Geometry check sheet. Reference: the model listing, model coordinates, mm. A direction names the side the tool comes from. Give positions to 0.01 mm unless a question says otherwise; leave off trailing zeros. Write each loop counter-clockwise with the first axis right and the second up, starting at its lowest first coordinate (ties: lowest second). Pieces come first, ordered by that corner, then holes.
(1) Cross-section at C-C (y = 1.25). Record the boundary of the cut face in (x, z).
(2) Mould release check, pull along Z, two halves, no side actions. Record for faces 1 (the flat face through (-2, 9, 5)), 2 (the cylindrical face through (-7.81, 12.99, -1.73)), 3 (the flat face through (-6, 0, 6)): +Z half, -Z half, draft (parallel to the pull), parting line (faces both ways), or undercut.
(3) Cross-section at B-B (z = 0). Record the boundary of the cut face in (x, y).
(4) Cross-section at A-A (x = 0). Record the boundary of the cut face in (y, z).
(5) Cross-section at D-D (x = 12.5). Record the boundary of the cut face in (y, z).
(6) Tool access check on faces 4 (the cylindrical face through (-4.88, 12.45, -1.08)), 5 (the cylindrical face through (-9.76, 14.49, -2.17)), 6 (the flat face through (8.2, 14, 0)), 7 (the cylindrical face through (0.33, 4.437, -7.493)). Record the directions out of +Z, -Z, +X, -X, +Y, -Y that give a thin tool (end or side, any length) a straight path to the whole face; none if there is none.
(7) Depth check by flat-ended pin: P1, Ø12, axis at x = -3.5, z = 1, coming from the -Y side; P2, Ø1.5, axis at x = 8.5, z = -9.5, coming from the +Y side; P3, Ø4, axis at x = 1, z = 1, coming from the -Y side; P4, Ø6, axis at y = 7.5, z = 9.5, coming from the -X side. Enter the tip coordinate at first touch or a pass-through.
(8) Thickness scan on line 1 along X through (y, z) = (11.5, 0); line 2 along X through (y, z) = (4, 0); line 3 along Y through (x, z) = (-2.5, -7.75). Record the ranges inside material, lowest first.
```python
from build123d import *

# Parameters (mm, degrees)
SKETCH_1_R           = 14.5
SKETCH_1_R_2         = 7.5
EXTRUDE_1_DEPTH      = 12
EXTRUDE_2_DEPTH      = 2
EXTRUDE_2_DEPTH_BACK = 3
SKETCH_2_R           = 8
SKETCH_2_R_2         = 5
SKETCH_3_R           = 10
SKETCH_3_R_2         = 5
EXTRUDE_3_DEPTH      = 2
FILLET_1_R           = 1


with BuildPart() as part:
    # Эскиз1 → Бобышка-Вытянуть1 (new body)
    with BuildSketch(Plane(origin=(0, 0, 0), x_dir=(1, 0, 0), z_dir=(0, 1, 0))):
        with Locations(Location((0, 0, 0), (0, 0, 270))):
            Circle(SKETCH_1_R)
        with Locations(Location((0, 0, 0), (0, 0, 270))):
            Circle(SKETCH_1_R_2, mode=Mode.SUBTRACT)
    extrude(amount=EXTRUDE_1_DEPTH)

    # Эскиз2 → Бобышка-Вытянуть2 (add, two sides: drawn at the far end of the back side and taken through both)
    with BuildSketch(Plane(origin=(0, 12, 0), x_dir=(1, 0, 0), z_dir=(0, 1, 0)).offset(-EXTRUDE_2_DEPTH_BACK)):
        with Locations(Location((0, 0, 0), (0, 0, 270))):
            Circle(SKETCH_2_R)
        with Locations(Location((0, 0, 0), (0, 0, 270))):
            Circle(SKETCH_2_R_2, mode=Mode.SUBTRACT)
    extrude(amount=EXTRUDE_2_DEPTH + EXTRUDE_2_DEPTH_BACK)

    # Эскиз3 → Бобышка-Вытянуть3 (add)
    with BuildSketch(Plane(origin=(0, 14, 0), x_dir=(1, 0, 0), z_dir=(0, 1, 0))):
        with Locations(Location((0, 0, 0), (0, 0, 270))):
            Circle(SKETCH_3_R)
        with Locations(Location((0, 0, 0), (0, 0, 270))):
            Circle(SKETCH_3_R_2, mode=Mode.SUBTRACT)
    extrude(amount=EXTRUDE_3_DEPTH)

    # Скругление1
    fillet_1_edges = [part.edges().sort_by_distance(p)[0] for p in [
        (0, 16, -10),
    ]]
    fillet(fillet_1_edges, radius=FILLET_1_R)


solid = part.part
```
Reply:
1. outline: circle Ø29 at (0, 0); hole circle Ø15 at (0, 0)
2. face 1: undercut
2. face 2: parting line
2. face 3: draft
3. outline: (-14.5, 0) - (-7.5, 0) - (-7.5, 9) - (-5, 9) - (-5, 16) - (-9, 16) arc R1 ccw to (-10, 15) - (-10, 14) - (-8, 14) - (-8, 12) - (-14.5, 12) - close; (5, 9) - (7.5, 9) - (7.5, 0) - (14.5, 0) - (14.5, 12) - (8, 12) - (8, 14) - (10, 14) - (10, 15) arc R1 ccw to (9, 16) - (5, 16) - close
4. outline: (0, -14.5) - (12, -14.5) - (12, -8) - (14, -8) - (14, -10) - (15, -10) arc R1 ccw to (16, -9) - (16, -5) - (9, -5) - (9, -7.5) - (0, -7.5) - close; (0, 7.5) - (9, 7.5) - (9, 5) - (16, 5) - (16, 9) arc R1 ccw to (15, 10) - (14, 10) - (14, 8) - (12, 8) - (12, 14.5) - (0, 14.5) - close
5. outline: (0, -7.35) - (12, -7.35) - (12, 7.35) - (0, 7.35) - close
6. face 4: +Y, -Y
6. face 5: +Y
6. face 6: none
6. face 7: -Y
7. P1: stops at y = 0
7. P2: stops at y = 12
7. P3: passes through
7. P4: stops at x = -12.96
8. line 1: x = -14.5 to -5, 5 to 14.5
8. line 2: x = -14.5 to -7.5, 7.5 to 14.5
8. line 3: y = 0 to 12, 14 to 16
